Autodesk Inventor part; units mm, degrees
ref_plane "YZ Plane" through (0, 0, 0) normal (1, 0, 0) x (0, 1, 0)
ref_plane "XZ Plane" through (0, 0, 0) normal (0, 1, 0) x (-1, 0, 0)
ref_plane "XY Plane" through (0, 0, 0) normal (0, 0, 1) x (1, 0, 0)
sketch "Sketch1" plane through (0, 0, 0) normal (0, 1, 0) x (-1, 0, 0)
  circle A0 centre (0, 0) radius 6.35
  dimension "d0" = 12.7
extrude "Extrusion1" add sketch "Sketch1" along normal blind 9.525
sketch "Sketch2" plane through (0, 9.525, 0) normal (0, 1, 0) x (1, 0, 0)
  line L0 (0, 7.3892) -> (6.3992, 3.6946)
  line L1 (6.3992, 3.6946) -> (6.3992, -3.6946)
  line L2 (6.3992, -3.6946) -> (0, -7.3892)
  line L3 (0, -7.3892) -> (-6.3992, -3.6946)
  line L4 (-6.3992, -3.6946) -> (-6.3992, 3.6946)
  line L5 (-6.3992, 3.6946) -> (0, 7.3892)
  point P0 (0, 0)
  point P1 (0, 0)
extrude "Extrusion2" add sketch "Sketch2" along normal blind 3.175
thread "Thread1"
sketch "Sketch3" plane through (0, 12.7, 0) normal (0, 1, 0) x (1, 0, 0)
  circle A0 centre (0, 0) radius 4.7625
  dimension "d7" = 9.525
extrude "Extrusion3" add sketch "Sketch3" along normal blind 3.175
sketch "Sketch4" plane through (0, 15.875, 0) normal (0, 1, 0) x (1, 0, 0)
  circle A0 centre (0, 0) radius 4.7625
  line L0 (6.3992, -10.3449) -> (6.3992, 10.3449)
revolve "Revolution1" add sketch "Sketch4" angle 90 about axis through (6.3992, 15.875, 3.6946) along (0, 0, -1)
sketch "Sketch5" plane through (6.3992, 22.2742, 0) normal (1, 0, 0) x (0, 0, -1)
  circle A0 centre (0, 0) radius 4.7625
  circle A1 centre (0, 0) radius 4.7625
  point P0 (0, -22.2742)
extrude "Extrusion4" add sketch "Sketch5" along normal blind 9.525
fillet "Fillet1" radius 3.175 1 edges at (15.9242, 22.2742, 4.7625)
sketch "Sketch6" plane through (15.9242, 22.2742, 0) normal (1, 0, 0) x (0, 0, -1)
  circle A0 centre (0, 0) radius 1.5875
  point P0 (0, -22.2742)
extrude "Extrusion5" cut sketch "Sketch6" against normal blind 9.525
sketch "Sketch7" plane through (0, 0, 0) normal (0, -1, 0) x (1, 0, 0)
  circle A0 centre (0, 0) radius 1.5875
  dimension "d16" = 3.175
extrude "Extrusion6" cut sketch "Sketch7" against normal blind 15.875
fillet "Fillet2" radius 1.27 1 edges at (6.35, 0, 0)
properties part number "Threaded Elbow"
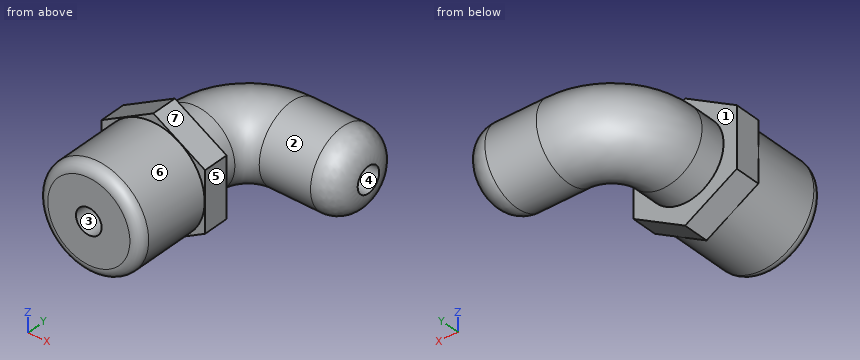
Read the model definition and answer for the solid it produces. Units are mm, in the model's axes. Face numbers are marked on the shaded views. A direction names the side the tool comes from. Give positions to 0.01 mm unless a question says otherwise; leave off trailing zeros. Write each loop counter-clockwise with the first axis right and the second up, starting at its lowest first coordinate (ties: lowest second). Pieces come first, ordered by that corner, then holes. Notation, with made-up numbers: (50, 30.5) -> (87, 30.5) arc R20 cw to (87, 52.5) -> close; hole circle Ø7 at (9.25, 86). An arc over 180 degrees is marked (long way). Answer in a Markdown table with one row per item.
1) Section A-A on y = 10 is taken. Give the vertices of the cut face in (x, z) (1 decimal).
Results list:
| item | result |
|---|---|
| outline | (-6.4, -3.7) -> (0, -7.4) -> (6.4, -3.7) -> (6.4, 3.7) -> (0, 7.4) -> (-6.4, 3.7) -> close; hole circle Ø3.2 at (0, 0) |
2) Each of these flat-tipped pins is pushed along its axis until it touches: pin 1 Ø3 at (x, z) = (0, 0) entering from +Y; pin 2 Ø1.9 at (y, z) = (22.27, 0) entering from -X; pin 3 Ø2 at (x, y) = (-2, 4) entering from -Z. Where does it stop, or does it pass through?
Results list:
| item | result |
|---|---|
| pin 1 | y = 25.9 |
| pin 2 | x = -3.34 |
| pin 3 | z = -6.27 |
3) A tool of negligible diameter and unlimited length cuts with its end or side. For the marked faces 5, 6 and 7, from which of +Z, -Z, +X, -X, +Y, -Y can it reach the whole face along a straight path? Write none if from no direction.
Results list:
| item | result |
|---|---|
| face 5 | +Z, -Z, +X, -Y |
| face 6 | -Y |
| face 7 | +Z, +X, -Y |
4) Section C-C on x = 10 is taken. Give the vertices of the cut face in (y, z) (1 decimal), plus the area to 3 significant figures.
Results list:
| item | result |
|---|---|
| outline | circle Ø9.5 at (22.3, 0); hole circle Ø3.2 at (22.3, 0) |
| area | 63.3 mm^2 |
5) Determine the mould class of the marked faces 1, 2, 3 and 4 for opening direction Z: released by +Z, released by -Z, zero draft, split by the parting line, or undercut.
Results list:
| item | result |
|---|---|
| face 1 | zero draft |
| face 2 | split by the parting line |
| face 3 | undercut |
| face 4 | undercut |
6) Straight lines are drawn through the part: line 1 (Z direction, x = 0, y = 5.5); line 2 (Y direction, x = 9.25, z = 0); line 3 (Z direction, x = 8.25, y = 23.25). For each, find the intervals that lie inside material, in ascending order. Write a range as [from, to].
Results list:
| item | result |
|---|---|
| line 1 | [-6.35, -1.59], [1.59, 6.35] |
| line 2 | [17.51, 20.69], [23.86, 27.04] |
| line 3 | [-4.66, -1.25], [1.25, 4.66] |
